Read the model definition and answer for the solid it produces. Units are mm, in the model's axes. A direction names the side the tool comes from. Coordinates: 2 decimals unless noted, no trailing zeros. Order: outer loops, then holes, each group sorted by start corner. A loop starts at its lowest first (then second) coordinate and runs counter-clockwise, first axis right, second up. Notation, with made-up numbers: (65, 74) -> (79, 74) arc R16 cw to (79, 103) -> close; hole circle Ø6 at (-5.5, -10.75). An arc over 180 degrees is marked (long way). Answer in a Markdown table with one row per item.
from build123d import *

# Parameters (mm, degrees)
F1_DEPTH = 790
F2_T     = -25


with BuildPart() as f1:
    # F0 (on Top) → F1 (new body)
    with BuildSketch(Plane.XY):
        Polygon((35.191152, -157.93012), (121.299235, -107.083311), (161.075133, -15.334316), (139.325805, 82.271865), (64.358755, 148.452991), (-35.191152, 157.93012), (-121.299235, 107.083311), (-161.075133, 15.334316), (-139.325805, -82.271865), (-64.358755, -148.452991), align=None)
    extrude(amount=F1_DEPTH)

    # F2
    f2_openings = [f1.faces().sort_by_distance(p)[0] for p in [
        (0, 0, 790),
    ]]
    offset(amount=F2_T, openings=f2_openings)


solid = f1.part
Q1. The part is cut by section C-C (y = 47). Write down the section's boundary in (x, z).
Outcome:
| item | result |
|---|---|
| outline | (-147.35, 0) -> (147.19, 0) -> (147.19, 790) -> (121.57, 790) -> (121.57, 25) -> (-120.1, 25) -> (-120.1, 790) -> (-147.35, 790) -> close |
Q2. For faces 5 (the face through (65.029, -111.278, 402.145)), 6 (the face through (-102.367, -114.899, 389.47)), determine the directions among +Z, -Z, +X, -X, +Y, -Y from which every point of the face is accessible in a straight line to the end or side of a thin tool.
Outcome:
| item | result |
|---|---|
| face 5 | +Z |
| face 6 | +Z, -Z, -X, -Y |
Q3. The part is cut by section B-B (x = -74). Write down the section's boundary in (y, z).
Outcome:
| item | result |
|---|---|
| outline | (-139.94, 0) -> (135.01, 0) -> (135.01, 790) -> (105.98, 790) -> (105.98, 25) -> (-106.59, 25) -> (-106.59, 790) -> (-139.94, 790) -> close |
Q4. The part is cut by section A-A (z = 587.5). Write down the section's boundary in (x, y).
Outcome:
| item | result |
|---|---|
| outline | (-161.08, 15.33) -> (-139.33, -82.27) -> (-64.36, -148.45) -> (35.19, -157.93) -> (121.3, -107.08) -> (161.08, -15.33) -> (139.33, 82.27) -> (64.36, 148.45) -> (-35.19, 157.93) -> (-121.3, 107.08) -> close; hole (-134.91, 12.84) -> (-116.69, -68.91) -> (-53.9, -124.34) -> (29.47, -132.27) -> (101.59, -89.69) -> (134.91, -12.84) -> (116.69, 68.91) -> (53.9, 124.34) -> (-29.47, 132.27) -> (-101.59, 89.69) -> close |
Q5. For a pull along Y with two mould halves and no side action, classify faces 1 (the face through (-77.642, 132.863, 389.47)), 2 (the face through (140.91, -61.85, 389.47)), 3 (the face through (125.926, 27.459, 402.145)), 4 (the face through (-118.02, 51.8, 402.14)) as pulls with the +Y half, pulls with the -Y half, needs draft (parallel to the pull), parting line crosses it, or undercut.
Outcome:
| item | result |
|---|---|
| face 1 | pulls with the +Y half |
| face 2 | pulls with the -Y half |
| face 3 | undercut |
| face 4 | undercut |
Q6. Consider line 1 (Z direction, x = 2, y = 129); line 2 (Y direction, x = 62, z = 72); line 3 (X direction, y = -88, z = 41). Determine where each line is inside the solid, lowest interval first.
Outcome:
| item | result |
|---|---|
| line 1 | 0 to 25 |
| line 2 | -142.1 to -113.07, 117.19 to 148.68 |
| line 3 | -132.84 to -95.06, 102.32 to 129.57 |
Q7. Given pin 1 (8 mm diameter, centred on y = 40, z = 548, fed in from -X); pin 2 (10 mm diameter, centred on x = 33.5, z = 113.5, fed in from -Y); pin 3 (8 mm diameter, centred on x = -48.5, z = 485, fed in from -Y), each flat-ended and moving along its own axis, determine where each tip first touches the part or whether it passes through.
Outcome:
| item | result |
|---|---|
| pin 1 | x = -152.12 |
| pin 2 | y = -157.93 |
| pin 3 | y = -150.34 |
